Geometry: final body of the model. Coordinates: model frame, mm. A direction names the side the tool comes from. Give positions to 0.01 mm unless a question says otherwise; leave off trailing zeros. Loops run counter-clockwise (first coordinate to the right, second up) from the corner with the lowest first, then second, coordinate; pieces in that order, holes last. Notation, with made-up numbers: (86.25, 41.5) -> (136.25, 41.5) arc R14 ccw to (136.25, 60.5) -> close; hole circle Ø7 at (-15.5, 57). An arc over 180 degrees is marked (long way). One line per item, written item: value. Start each with the question number.
from build123d import *

# Parameters (mm, degrees)
SKETCH1_R                            = 75
BOSS_EXTRUDE1_DEPTH                  = 5
BOSS_EXTRUDE2_REACH                  = 108.184
BOSS_EXTRUDE2_END_RADIUS             = 75
BOSS_EXTRUDE2_DIRECTION_2_REACH      = 108.184
BOSS_EXTRUDE2_DIRECTION_2_END_RADIUS = 75
SKETCH3_R                            = 9.5
CUT_EXTRUDE1_DEPTH                   = 107.742681248
SKETCH4_R                            = 2
CUT_EXTRUDE2_DEPTH                   = 107.742681248


with BuildPart() as part:
    # Sketch1 → Boss-Extrude1 (new body)
    with BuildSketch(Plane(origin=(0, 0, 0), x_dir=(1, 0, 0), z_dir=(0, 1, 0))):
        with Locations(Location((0, 0, 0), (0, 0, 270))):
            Circle(SKETCH1_R)
    extrude(amount=BOSS_EXTRUDE1_DEPTH)

    # Boss-Extrude2: up to this cylinder (the profile starts inside it)
    boss_extrude2_end = Plane(origin=(0, 12, 0), z_dir=(0, -1, 0)) * Cylinder(BOSS_EXTRUDE2_END_RADIUS, 373.368, mode=Mode.PRIVATE)
    # Sketch2 → Boss-Extrude2 (add, up to the surface)
    with BuildSketch(Plane.XY, mode=Mode.PRIVATE) as boss_extrude2_sk1:
        Polygon((-15, 5), (-15, 13), (-8, 13), (-8, 17), (-19, 17), (-19, 5), align=None)
    boss_extrude2_tool1 = extrude(boss_extrude2_sk1.sketch, amount=BOSS_EXTRUDE2_REACH, mode=Mode.PRIVATE) & boss_extrude2_end
    add(boss_extrude2_tool1.solids().sort_by_distance((-15.162788, 9, 0))[0])
    # Sketch2 → Boss-Extrude2 (add, up to the surface)
    with BuildSketch(Plane.XY, mode=Mode.PRIVATE) as boss_extrude2_sk2:
        Polygon((8, 17), (8, 13), (15, 13), (15, 5), (19, 5), (19, 17), align=None)
    boss_extrude2_tool2 = extrude(boss_extrude2_sk2.sketch, amount=BOSS_EXTRUDE2_REACH, mode=Mode.PRIVATE) & boss_extrude2_end
    add(boss_extrude2_tool2.solids().sort_by_distance((8.162788, 15, 0))[0])

    # Boss-Extrude2 direction 2: up to this cylinder (the profile starts inside it)
    boss_extrude2_direction_2_end = Plane(origin=(0, 12, 0), z_dir=(0, -1, 0)) * Cylinder(BOSS_EXTRUDE2_DIRECTION_2_END_RADIUS, 373.368, mode=Mode.PRIVATE)
    # Sketch2 → Boss-Extrude2 direction 2 (add, up to the surface)
    with BuildSketch(Plane.XY, mode=Mode.PRIVATE) as boss_extrude2_direction_2_sk1:
        Polygon((-15, 5), (-15, 13), (-8, 13), (-8, 17), (-19, 17), (-19, 5), align=None)
    boss_extrude2_direction_2_tool1 = extrude(boss_extrude2_direction_2_sk1.sketch, amount=-BOSS_EXTRUDE2_DIRECTION_2_REACH, mode=Mode.PRIVATE) & boss_extrude2_direction_2_end
    add(boss_extrude2_direction_2_tool1.solids().sort_by_distance((-15.162788, 9, 0))[0])
    # Sketch2 → Boss-Extrude2 direction 2 (add, up to the surface)
    with BuildSketch(Plane.XY, mode=Mode.PRIVATE) as boss_extrude2_direction_2_sk2:
        Polygon((8, 17), (8, 13), (15, 13), (15, 5), (19, 5), (19, 17), align=None)
    boss_extrude2_direction_2_tool2 = extrude(boss_extrude2_direction_2_sk2.sketch, amount=-BOSS_EXTRUDE2_DIRECTION_2_REACH, mode=Mode.PRIVATE) & boss_extrude2_direction_2_end
    add(boss_extrude2_direction_2_tool2.solids().sort_by_distance((8.162788, 15, 0))[0])

    # Sketch3 → Cut-Extrude1 (cut, through all)
    with BuildSketch(Plane(origin=(0, 5, 0), x_dir=(1, 0, 0), z_dir=(0, 1, 0))):
        with Locations(Location((0, 0, 0), (0, 0, 270))):
            Circle(SKETCH3_R)
    extrude(amount=-CUT_EXTRUDE1_DEPTH, mode=Mode.SUBTRACT)

    # Sketch4 → Cut-Extrude2 (cut, through all)
    with BuildSketch(Plane(origin=(0, 5, 0), x_dir=(1, 0, 0), z_dir=(0, 1, 0))):
        with Locations(Location((-45, 35, 0), (0, 0, 270))):
            Circle(SKETCH4_R)
        with Locations(Location((45, 35, 0), (0, 0, 270))):
            Circle(SKETCH4_R)
        with Locations(Location((45, -35, 0), (0, 0, 270))):
            Circle(SKETCH4_R)
        with Locations(Location((-45, -35, 0), (0, 0, 270))):
            Circle(SKETCH4_R)
    extrude(amount=-CUT_EXTRUDE2_DEPTH, mode=Mode.SUBTRACT)


solid = part.part
Item 1: Pin query (flat end, axial travel): pin 1 (9.5 mm diameter, centred on y = 8, z = 36, fed in from -X); pin 2 (2 mm diameter, centred on x = 4, z = 18, fed in from -Y); pin 3 (3.5 mm diameter, centred on y = 8.5, z = 19.5, fed in from +X); pin 4 (5 mm diameter, centred on y = 5, z = 27.5, fed in from -X). Return the tip coordinate at first contact, or that it passes through.
Item 2: Access query for faces 4 (the face through (41, 5, -1)), 5 (the face through (-5.78, 2.54, -7.54)), 6 (the face through (15, 9, 1)), 7 (the face through (8, 15, 1)). Directions: +Z, -Z, +X, -X, +Y, -Y. A direction counts if a zero-diameter tool reaches every point of the face in a straight line with its end or side. Return the directions, or none.
Item 3: Section C-C, the plane z = -45. Output: boundary loops of the cut face in (x, y).
Item 4: Mould query, pull axis X, two halves, no side actions, for faces 1 (the face through (-13, 17, 1)), 2 (the face through (-19, 11, 1)), 3 (the face through (-8, 15, 1)). Classes: pulls with the +X half, pulls with the -X half, needs draft (parallel to the pull), parting line crosses it, or undercut.
Item 5: Section A-A, the plane x = -45. Output: boundary loops of the cut face in (y, z), then the cut area to 3 significant figures.
Item 6: Section B-B, the plane y = 15.25. Output: boundary loops of the cut face in (x, z).
Item 7: Section D-D, the plane z = 35. Output: boundary loops of the cut face in (x, y), then the cut area to 3 significant figures.
Item 8: Ray query, line 1 along Y through (x, z) = (14.5, -30.5); line 2 along X through (y, z) = (15.25, -8.5); line 3 along X through (y, z) = (2.65, 35). Return the intervals inside material, ascending. Write a range as [from, to].
Geometry check:
1. pin 1: stops at x = -67.68
1. pin 2: stops at y = 0
1. pin 3: stops at x = 19
1. pin 4: stops at x = -70.71
2. face 4: +Z, -Z, +X, +Y
2. face 5: -Y
2. face 6: +Z, -Z
2. face 7: +Z, -Z, +Y
3. outline: (-60, 0) -> (60, 0) -> (60, 5) -> (19, 5) -> (19, 17) -> (8, 17) -> (8, 13) -> (15, 13) -> (15, 5) -> (-15, 5) -> (-15, 13) -> (-8, 13) -> (-8, 17) -> (-19, 17) -> (-19, 5) -> (-60, 5) -> close
4. face 1: needs draft
4. face 2: pulls with the -X half
4. face 3: undercut
5. outline: (0, -60) -> (5, -60) -> (5, -37) -> (0, -37) -> close; (0, -33) -> (5, -33) -> (5, 33) -> (0, 33) -> close; (0, 37) -> (5, 37) -> (5, 60) -> (0, 60) -> close
5. area: 560 mm2
6. outline: (-19, -72.55) arc R75 ccw to (-8, -74.57) -> (-8, 74.57) arc R75 ccw to (-19, 72.55) -> close; (8, -74.57) arc R75 ccw to (19, -72.55) -> (19, 72.55) arc R75 ccw to (8, 74.57) -> close
7. outline: (-66.33, 0) -> (-47, 0) -> (-47, 5) -> (-66.33, 5) -> close; (-43, 0) -> (43, 0) -> (43, 5) -> (19, 5) -> (19, 17) -> (8, 17) -> (8, 13) -> (15, 13) -> (15, 5) -> (-15, 5) -> (-15, 13) -> (-8, 13) -> (-8, 17) -> (-19, 17) -> (-19, 5) -> (-43, 5) -> close; (47, 0) -> (66.33, 0) -> (66.33, 5) -> (47, 5) -> close
7. area: 775 mm2
8. line 1: y = [0, 5], [13, 17]
8. line 2: x = [-19, -8], [8, 19]
8. line 3: x = [-66.33, -47], [-43, 43], [47, 66.33]
